```python
from build123d import *

# Parameters (mm, degrees)
SKETCH1_W           = 25.4
SKETCH1_H           = 9.525
BOSS_EXTRUDE1_DEPTH = 100.076
SKETCH2_R           = 3.3734375
SKETCH2_R_2         = 9.498
CUT_EXTRUDE1_DEPTH  = 102.3272984


with BuildPart() as part:
    # Sketch1 → Boss-Extrude1 (new body)
    with BuildSketch(Plane.XY):
        Rectangle(SKETCH1_W, SKETCH1_H)
    extrude(amount=BOSS_EXTRUDE1_DEPTH)

    # Sketch2 → Cut-Extrude1 (cut, through all)
    with BuildSketch(Plane(origin=(0, 4.7625, 0), x_dir=(1, 0, 0), z_dir=(0, 1, 0))):
        with Locations(Location((0, -16.0734375, 0), (0, 0, 180))):
            Circle(SKETCH2_R)
        with Locations(Location((0, -41.4734375, 0), (0, 0, 180))):
            Circle(SKETCH2_R)
        with Locations(Location((0, -66.8734375, 0), (0, 0, 180))):
            Circle(SKETCH2_R_2)
    extrude(amount=-CUT_EXTRUDE1_DEPTH, mode=Mode.SUBTRACT)


solid = part.part
```
Check sheet for the modelled part. Datum: model origin and axes. Units: mm. Give positions to 0.01 mm unless a question says otherwise; leave off trailing zeros. Write each loop counter-clockwise with the first axis right and the second up, starting at its lowest first coordinate (ties: lowest second). Pieces come first, ordered by that corner, then holes.
Item 1: Scan lines: L1, parallel to Z at x = 0, y = 2.75; L2, parallel to Z at x = 6, y = -1.75; L3, parallel to Z at x = 8, y = -1.5. Record each from-to range of solid material in increasing order.
Item 2: Cross-section at B-B (x = -6.75). Enter the section's corners in (y, z).
Item 3: Cross-section at C-C (z = 62). Enter the section's corners in (x, y).
Item 4: Draft check along Z on faces 1 (the face through (0.73, 0.07, 38.18)), 2 (the face through (0, -4.762, 49)), 3 (the face through (0, 0, 100.076)). Enter one of: released by +Z, released by -Z, zero draft, split by the parting line, or undercut.
Item 5: Cross-section at D-D (y = 0.75). Enter the section's corners in (x, z).
Item 6: Cross-section at A-A (x = 0). Enter the section's corners in (y, z).
Report:
1. L1: z = 0 to 12.7, 19.45 to 38.1, 44.85 to 57.38, 76.37 to 100.08
1. L2: z = 0 to 59.51, 74.24 to 100.08
1. L3: z = 0 to 61.75, 71.99 to 100.08
2. outline: (-4.76, 0) - (4.76, 0) - (4.76, 60.19) - (-4.76, 60.19) - close; (-4.76, 73.56) - (4.76, 73.56) - (4.76, 100.08) - (-4.76, 100.08) - close
3. outline: (-12.7, -4.76) - (-8.15, -4.76) - (-8.15, 4.76) - (-12.7, 4.76) - close; (8.15, -4.76) - (12.7, -4.76) - (12.7, 4.76) - (8.15, 4.76) - close
4. face 1: undercut
4. face 2: zero draft
4. face 3: released by +Z
5. outline: (-12.7, 0) - (12.7, 0) - (12.7, 100.08) - (-12.7, 100.08) - close; hole circle Ø19 at (0, 66.87); hole circle Ø6.75 at (0, 16.07); hole circle Ø6.75 at (0, 41.47)
6. outline: (-4.76, 0) - (4.76, 0) - (4.76, 12.7) - (-4.76, 12.7) - close; (-4.76, 19.45) - (4.76, 19.45) - (4.76, 38.1) - (-4.76, 38.1) - close; (-4.76, 44.85) - (4.76, 44.85) - (4.76, 57.38) - (-4.76, 57.38) - close; (-4.76, 76.37) - (4.76, 76.37) - (4.76, 100.08) - (-4.76, 100.08) - close
